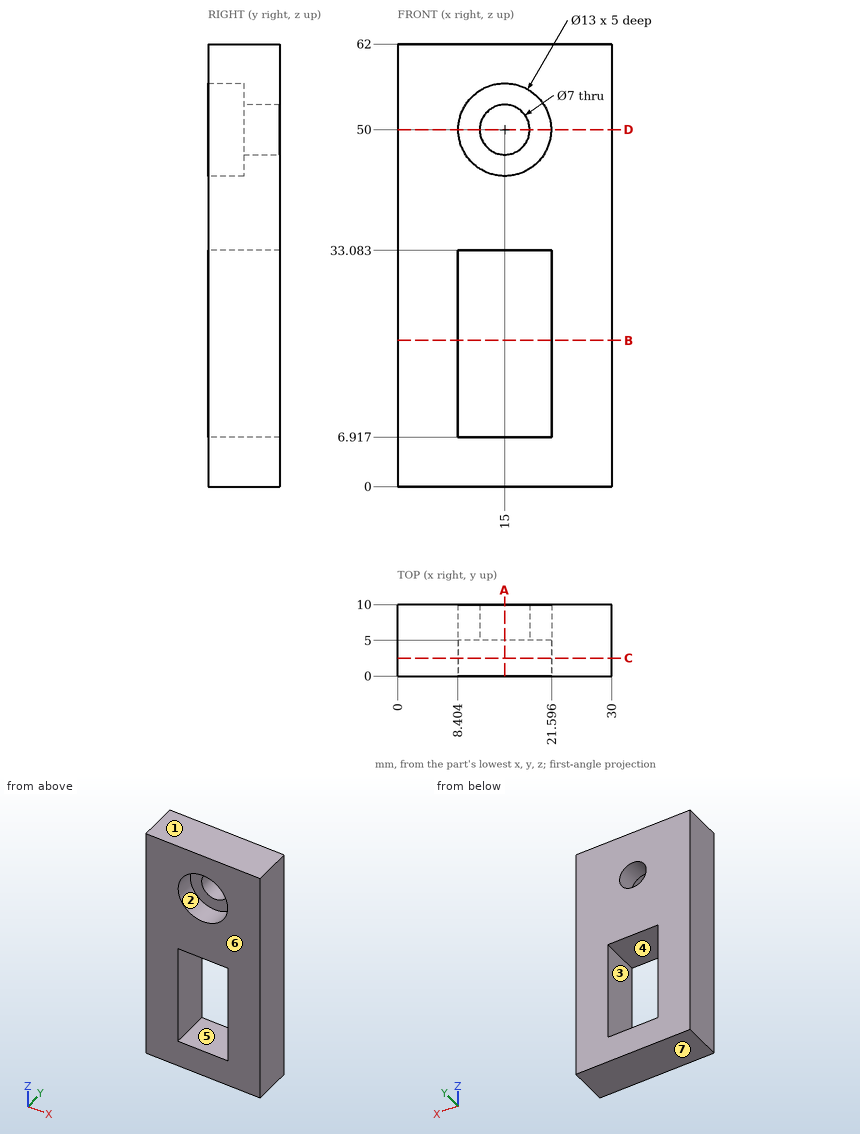
Answer from the drawing. Dimensions are ordinates in mm from the lowest x, y and z of the part. A direction names the side the tool comes from. Give positions to 0.01 mm unless a question says otherwise; leave off trailing zeros. Loops run counter-clockwise (first coordinate to the right, second up) from the corner with the lowest first, then second, coordinate; pieces in that order, holes last. Notation, with made-up numbers: (-33.5, -16) -> (13.5, -16) arc R13 ccw to (13.5, -10) -> close; hole circle Ø2 at (39.5, 45). An arc over 180 degrees is marked (long way). Answer as CSV lines item,"result".
Item 1: Find section B-B on z = 20.5. Give the vertices of the cut face in (x, y), plus the area to 3 significant figures.
Returned:
outline,"(0, 0) -> (8.4, 0) -> (8.4, 10) -> (0, 10) -> close; (21.6, 0) -> (30, 0) -> (30, 10) -> (21.6, 10) -> close"
area,"168 mm²"
Item 2: Consider line 1 (Z direction, x = 10.5, y = 5.5); line 2 (X direction, y = 3.1, z = 50); line 3 (X direction, y = 3.25, z = 29). Determine where each line is inside the solid, lowest interval first. Write a range as [from, to].
Returned:
line 1,"z = [0, 6.92], [33.08, 62]"
line 2,"x = [0, 8.5], [21.5, 30]"
line 3,"x = [0, 8.4], [21.6, 30]"
Item 3: Find section C-C on y = 2.5. Give the vertices of the cut face in (x, z).
Returned:
outline,"(0, 0) -> (30, 0) -> (30, 62) -> (0, 62) -> close; hole (8.4, 6.92) -> (21.6, 6.92) -> (21.6, 33.08) -> (8.4, 33.08) -> close; hole circle Ø13 at (15, 50)"
Item 4: For the marked faces 1, 2 and 3, determine the directions among +Z, -Z, +X, -X, +Y, -Y from which every point of the face is accessible in a straight line to the end or side of a thin tool.
Returned:
face 1,"+Z, +X, -X, +Y, -Y"
face 2,"-Y"
face 3,"+Y, -Y"
Item 5: Find section D-D on z = 50. Give the vertices of the cut face in (x, y).
Returned:
outline,"(0, 0) -> (8.5, 0) -> (8.5, 5) -> (11.5, 5) -> (11.5, 10) -> (0, 10) -> close; (18.5, 5) -> (21.5, 5) -> (21.5, 0) -> (30, 0) -> (30, 10) -> (18.5, 10) -> close"
Item 6: Determine the mould class of the marked faces 4, 5, 6 and 7 for opening direction Z: +Z half, -Z half, draft (parallel to the pull), parting line (faces both ways), or undercut.
Returned:
face 4,"undercut"
face 5,"undercut"
face 6,"draft"
face 7,"-Z half"
Item 7: Find section A-A on x = 15. Give the vertices of the cut face in (y, z).
Returned:
outline,"(0, 0) -> (10, 0) -> (10, 6.92) -> (0, 6.92) -> close; (0, 33.08) -> (10, 33.08) -> (10, 46.5) -> (5, 46.5) -> (5, 43.5) -> (0, 43.5) -> close; (0, 56.5) -> (5, 56.5) -> (5, 53.5) -> (10, 53.5) -> (10, 62) -> (0, 62) -> close"
Item 8: Each of these flat-tipped pins is pushed along its axis until it touches: pin 1 (3 mm diameter, centred on y = 4, z = 15.5, fed in from -X); pin 2 (10.5 mm diameter, centred on x = 15, z = 50, fed in from -Y). Where does it stop, or does it pass through?
Returned:
pin 1,"stops at x = 0"
pin 2,"stops at y = 5"
